Design review of the part built by this model. Coordinates are the model's own, in mm. A direction names the side the tool comes from. Give positions to 0.01 mm unless a question says otherwise; leave off trailing zeros. Write each loop counter-clockwise with the first axis right and the second up, starting at its lowest first coordinate (ties: lowest second). Pieces come first, ordered by that corner, then holes. Notation, with made-up numbers: M 66.25,64 L 122.25,64 A24 ccw 122.25,83 Z; hole C 77,-34 d3. An arc over 180 degrees is marked long. Answer in a Markdown table with one row per item.
```python
from build123d import *

# Parameters (mm, degrees)
CUT_EXTRUDE1_DEPTH      = 43.532340636
CUT_EXTRUDE1_DEPTH_BACK = 43.532340636
SKETCH2_W               = 2.4
SKETCH2_H               = 2.4


with BuildPart() as part:
    # Sketch1 → Revolve1 (revolve)
    with BuildSketch(Plane.XY, mode=Mode.PRIVATE) as revolve1_sk:
        Polygon((0, 0), (6, 6), (6, 33), (12, 39), (0, 39), align=None)
    revolve(revolve1_sk.sketch.rotate(Axis((0, 39, 0), (0, -1, 0)), 180), axis=Axis((0, 39, 0), (0, -1, 0)))

    # Sketch2 → Cut-Extrude1 (cut, two sides: drawn at the far end of the back side and taken through both)
    with BuildSketch(Plane.XY.offset(-CUT_EXTRUDE1_DEPTH_BACK)):
        with Locations((0, 37.8)):
            Rectangle(SKETCH2_W, SKETCH2_H)
    extrude(amount=CUT_EXTRUDE1_DEPTH + CUT_EXTRUDE1_DEPTH_BACK, mode=Mode.SUBTRACT)


solid = part.part
```
1) Add section B-B (y = 35). Write out the cut boundary in (x, z).
Geometry says:
| item | result |
|---|---|
| outline | C 0,0 d16 |
2) The part is to be moulded in two halves that separate along X. For faces 3 (the face through (-5.723, 19.689, -1.802)), 4 (the face through (-5, 39, 0)), 5 (the face through (1.2, 38, 0)), 6 (the face through (0, 36.6, 0)), say which applies: released by +X, released by -X, zero draft, split by the parting line, or undercut.
Geometry says:
| item | result |
|---|---|
| face 3 | split by the parting line |
| face 4 | zero draft |
| face 5 | undercut |
| face 6 | undercut |
3) Add section A-A (y = 11). Write out the cut boundary in (x, z), and give its area (3 significant figures).
Geometry says:
| item | result |
|---|---|
| outline | C 0,0 d12 |
| area | 113 mm^2 |
4) For faces 1 (the face through (-1.2, 38, 0)), 2 (the face through (-0.8, 1.7, 1.5)), list the 3-axis set-ups (+Z, -Z, +X, -X, +Y, -Y) from which the entire face can be reached by the end or side of a thin tool; tool diameter is ignored.
Geometry says:
| item | result |
|---|---|
| face 1 | +Z, -Z, +Y |
| face 2 | -Y |
5) To check wall thickness, follow probe 1 along Z at (x, y) = (0.25, 24.5); probe 2 along X at (y, z) = (23.5, -5); probe 3 along Y at (x, z) = (5.25, 3.5). State the ranges of each line that lie inside material, in increasing order. Write a range as [from, to].
Geometry says:
| item | result |
|---|---|
| probe 1 | [-5.99, 5.99] |
| probe 2 | [-3.32, 3.32] |
| probe 3 | [33.31, 39] |
6) Insertion check: P1, Ø0.7, axis at y = 38, z = 4, coming from the -X side; P2, Ø6, axis at x = 0, y = 8, coming from the +Z side; P3, Ø8, axis at x = 3.5, y = 25.5, coming from the -Z side. Each pin has a flat end and moves straight along its axis. Give the tip position at first contact, or say it passes through.
Geometry says:
| item | result |
|---|---|
| P1 | x = -10.64 |
| P2 | z = 6 |
| P3 | z = -6 |
